Could you check a few things on this model? Use its own coordinates, in mm. Face numbers are marked on the shaded views. A direction names the side the tool comes from. Give positions to 0.01 mm unless a question says otherwise; leave off trailing zeros. Loops run counter-clockwise (first coordinate to the right, second up) from the corner with the lowest first, then second, coordinate; pieces in that order, holes last. Notation, with made-up numbers: M 60.25,74 L 74.25,74 A21 cw 74.25,86 Z; hole C 19,89 d8. An arc over 180 degrees is marked long. Use CSV: the item, a comma, the result in double quotes.
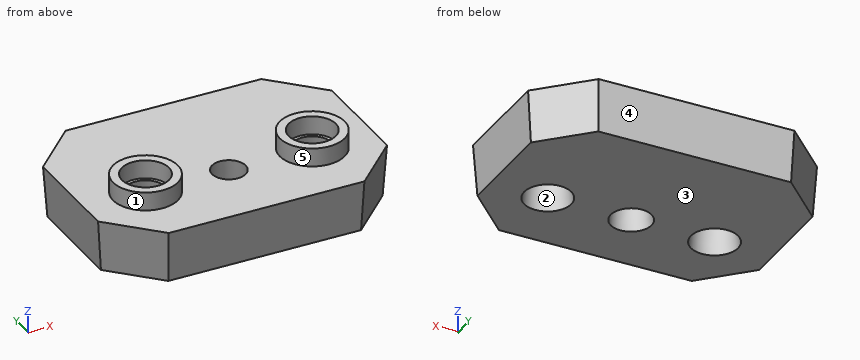
```python
from build123d import *

# Parameters (mm, degrees)
SKETCH1_R           = 12.7
SKETCH1_R_2         = 11
BOSS_EXTRUDE1_DEPTH = 28
BOSS_EXTRUDE1_DRAFT = -4
SKETCH2_R           = 17.5
SKETCH2_R_2         = 12.7
BOSS_EXTRUDE2_DEPTH = 38


with BuildPart() as part:
    # Sketch1 → Boss-Extrude1 (with draft: the straight prism first)
    with BuildSketch(Plane.XY):
        Polygon((-52, 52), (-76, 28), (-76, -28), (-52, -52), (52, -52), (76, -28), (76, 28), (52, 52), align=None)
        with Locations((-45, -14.5)):
            Circle(SKETCH1_R, mode=Mode.SUBTRACT)
        with Locations((45, -14.5)):
            Circle(SKETCH1_R, mode=Mode.SUBTRACT)
        with Locations((0, -14.5)):
            Circle(SKETCH1_R_2, mode=Mode.SUBTRACT)
    extrude(amount=BOSS_EXTRUDE1_DEPTH)
    # Boss-Extrude1: the draft: its side faces are tilted about the plane it starts from
    boss_extrude1_sides = [part.faces().sort_by_distance(p)[0] for p in [
        (-64, 40, 14),
        (-76, 0, 14),
        (-64, -40, 14),
        (0, -52, 14),
        (64, -40, 14),
        (76, 0, 14),
        (64, 40, 14),
        (0, 52, 14),
        (-57.7, -14.5, 14),
        (32.3, -14.5, 14),
        (-11, -14.5, 14),
    ]]
    draft(boss_extrude1_sides, Plane.XY, BOSS_EXTRUDE1_DRAFT)

    # Sketch2 → Boss-Extrude2 (add)
    # profile 1 of 2: a face of its own
    with BuildSketch(Plane.XY):
        with Locations(Location((-45, -14.5, 0), (0, 0, 180))):
            Circle(SKETCH2_R)
        with Locations(Location((-45, -14.5, 0), (0, 0, 180))):
            Circle(SKETCH2_R_2, mode=Mode.SUBTRACT)
    # profile 2 of 2: a face of its own
    with BuildSketch(Plane.XY):
        with Locations(Location((45, -14.5, 0), (0, 0, 180))):
            Circle(SKETCH2_R)
        with Locations(Location((45, -14.5, 0), (0, 0, 180))):
            Circle(SKETCH2_R_2, mode=Mode.SUBTRACT)
    extrude(amount=BOSS_EXTRUDE2_DEPTH)


solid = part.part
```
1. I want a section at B-B, the plane z = 33. List the corners of the cut face in (x, y) for me.
Outcome:
outline,"C -45,-14.5 d35; C 45,-14.5 d35; hole C -45,-14.5 d25.4; hole C 45,-14.5 d25.4"
2. I want a section at C-C, the plane y = -14.5. Give the number of separate pieces and of enclosed holes in the cut face, then the cut area to 3 significant figures.
Outcome:
separate pieces,"4"
enclosed holes,"0"
area,"2,630 mm2"
3. I'm going to push flat-ended pins straight in: pin 1 Ø2 at (x, z) = (41.5, 5) entering from -Y; pin 2 Ø5 at (x, z) = (-19.5, 15) entering from -Y; pin 3 Ø1 at (y, z) = (-28.5, 20) entering from -X; pin 4 Ø7.5 at (x, y) = (50, -17.5) entering from +Z. Where does each tip first touch, or does it pass through?
Outcome:
pin 1,"y = -52.42"
pin 2,"y = -53.22"
pin 3,"x = -77.43"
pin 4,"through"
4. I want a section at A-A, the plane z = 3.5. List the corners of the cut face in (x, y) for me.
Outcome:
outline,"M -76.24,-28.1 L -52.1,-52.24 L 52.1,-52.24 L 76.24,-28.1 L 76.24,28.1 L 52.1,52.24 L -52.1,52.24 L -76.24,28.1 Z; hole C -45,-14.5 d24.91; hole C 0,-14.5 d21.51; hole C 45,-14.5 d24.91"
5. Which directions (+Z, -Z, +X, -X, +Y, -Y) give clear straight access to the entire face, cutting with the end or side of a thin tool? Please do the marked faces 4 and 5.
Outcome:
face 4,"-Z, +X, -X, +Y"
face 5,"+Z"
6. If we mould it in two halves opening along Y, with no side actions, what happens to the marked faces 1, 2 and 3? For each: +Y half, -Y half, draft (parallel to the pull), parting line (faces both ways), or undercut.
Outcome:
face 1,"parting line"
face 2,"undercut"
face 3,"draft"
7. Please list where these lines run through material, in increasing order: line 1 (Y direction, x = 45, z = 33.5); line 2 (Z direction, x = -26.5, y = -7); line 3 (X direction, y = -7, z = 17).
Outcome:
line 1,"-32 to -27.2, -1.8 to 3"
line 2,"0 to 28"
line 3,"-77.19 to -53.73, -36.27 to -6.33, 6.33 to 36.27, 53.73 to 77.19"
8. I want a section at D-D, the plane x = 45. List the corners of the cut face in (y, z) for me, then the cut area to 3 significant figures.
Outcome:
outline,"M -53.96,28 L -52,0 L -27.2,0 L -25.24,28 L -27.2,28 L -27.2,38 L -32,38 L -32,28 Z; M -3.76,28 L -1.8,0 L 52,0 L 53.96,28 L 3,28 L 3,38 L -1.8,38 L -1.8,28 Z"
area,"2,410 mm2"
